Answer from the drawing. Dimensions are ordinates in mm from the lowest x, y and z of the part. A direction names the side the tool comes from. Give positions to 0.01 mm unless a question says otherwise; leave off trailing zeros. Loops run counter-clockwise (first coordinate to the right, second up) from the corner with the lowest first, then second, coordinate; pieces in that order, holes last.
(1) Which of the six approach directions +Z, -Z, +X, -X, +Y, -Y give full straight-line access (tool end or side, diameter ignored) to the marked faces 1, 2, 3 and 4?
(2) Find section D-D, the plane x = 14. Write down the section's boundary in (y, z).
(3) Find section C-C, the plane y = 21.75. Write down the section's boundary in (x, z) (1 decimal).
(4) Each of these flat-tipped pins is pushed along its axis until it touches: P1, Ø10, axis at x = 9, y = 15, coming from the -Z side; P2, Ø1.5, axis at y = 5, z = 15, coming from the +X side; P3, Ø1.5, axis at x = 35, y = 14, coming from the -Z side; P4, Ø2, axis at x = 9, y = 26, coming from the +Z side. Where does it stop, or does it pass through?
(5) Find section B-B, the plane z = 23.9. Write down the section's boundary in (x, y).
(6) Straight lines are drawn through the part: probe 1 along X at (y, z) = (17.5, 45.7); probe 2 along X at (y, z) = (16, 23.9); probe 3 along Z at (x, y) = (45, 21.5). For each, find the intervals that lie inside material, in ascending order.
(7) Determine the mould class of the marked faces 5, 6, 7 and 8 for opening direction Z: pulls with the +Z half, pulls with the -Z half, needs draft (parallel to the pull), parting line crosses it, or undercut.
(8) Find section A-A, the plane x = 44. Write down the section's boundary in (y, z), then the cut area to 3 significant figures.
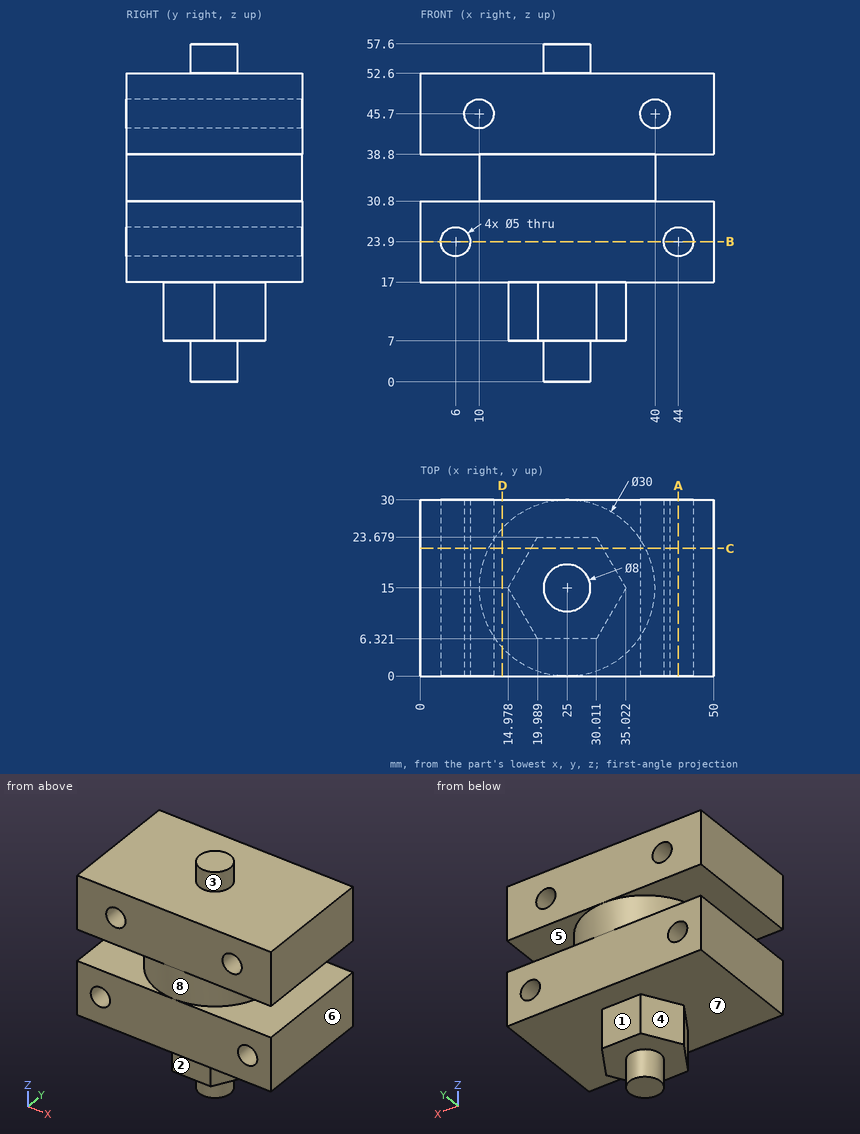
Entries:
1. face 1: -Z, +X, -X, +Y
1. face 2: -Z, +X, -X, -Y
1. face 3: +Z
1. face 4: -Z, -X, +Y
2. outline: (0, 17) - (30, 17) - (30, 30.8) - (25.2, 30.8) - (25.2, 38.8) - (30, 38.8) - (30, 52.6) - (0, 52.6) - (0, 38.8) - (4.8, 38.8) - (4.8, 30.8) - (0, 30.8) - close
3. outline: (0, 17) - (18.9, 17) - (18.9, 7) - (31.1, 7) - (31.1, 17) - (50, 17) - (50, 30.8) - (38.4, 30.8) - (38.4, 38.8) - (50, 38.8) - (50, 52.6) - (0, 52.6) - (0, 38.8) - (11.6, 38.8) - (11.6, 30.8) - (0, 30.8) - close; hole circle Ø5 at (6, 23.9); hole circle Ø5 at (10, 45.7); hole circle Ø5 at (40, 45.7); hole circle Ø5 at (44, 23.9)
4. P1: stops at z = 17
4. P2: passes through
4. P3: stops at z = 7
4. P4: stops at z = 52.6
5. outline: (0, 0) - (3.5, 0) - (3.5, 30) - (0, 30) - close; (8.5, 0) - (41.5, 0) - (41.5, 30) - (8.5, 30) - close; (46.5, 0) - (50, 0) - (50, 30) - (46.5, 30) - close
6. probe 1: x = 0 to 7.5, 12.5 to 37.5, 42.5 to 50
6. probe 2: x = 0 to 3.5, 8.5 to 41.5, 46.5 to 50
6. probe 3: z = 17 to 21.61, 26.19 to 30.8, 38.8 to 52.6
7. face 5: undercut
7. face 6: needs draft
7. face 7: pulls with the -Z half
7. face 8: undercut
8. outline: (0, 17) - (30, 17) - (30, 21.4) - (0, 21.4) - close; (0, 26.4) - (30, 26.4) - (30, 30.8) - (0, 30.8) - close; (0, 38.8) - (30, 38.8) - (30, 52.6) - (0, 52.6) - close
8. area: 678 mm2
